Read the model definition and answer for the solid it produces. Units are mm, in the model's axes. A direction names the side the tool comes from. Coordinates: 2 decimals unless noted, no trailing zeros. Write each loop counter-clockwise with the first axis right and the second up, starting at its lowest first coordinate (ties: lowest second). Pieces come first, ordered by that corner, then holes. Notation, with made-up numbers: (79.5, 77.25) -> (116.5, 77.25) arc R24 cw to (116.5, 113.25) -> close; hole circle Ø8 at (2.25, 66). An arc over 180 degrees is marked (long way). Write item = value, one per line. Start each with the question number.
1) A tool of negligible diameter and unlimited length cuts with its end or side. For faces 5 (the face through (-45, 2, 35.813)), 6 (the face through (-41.221, 2, 18)), 7 (the face through (-32.721, 3, 27)), from which of +Z, -Z, +X, -X, +Y, -Y can it reach the whole face along a straight path? Write none if from no direction.
2) Section A-A (y = 1.3) is taken. Determine the outline of the cut face in (x, z), plus the area to 3 significant figures.
3) For a pull along Z with two mould halves and no side action, classify faces 1 (the face through (-41, 3.5, 34)), 2 (the face through (-45, 2, 36.813)), 3 (the face through (-36, 2, 17.613)), 4 (the face through (-32.221, 2, 27)) as released by +Z, released by -Z, zero draft, split by the parting line, or undercut.
4) Flat-ended cylindrical pins translate along their axes: pin 1 Ø1.1 at (y, z) = (3, 27) entering from -X; pin 2 Ø1.2 at (y, z) = (1, 18) entering from -X; pin 3 Ø1 at (x, y) = (-48, 1) entering from -Z. Find the tip coordinate at first contact, or state that the pin passes through.
5) Section B-B (z = 30.75) is taken. Determine the outline of the cut face in (x, y).
6) Find the intervals of material crossed by line 1 along X through (y, z) = (2.85, 26.5); line 2 along X through (y, z) = (2.45, 33); line 3 along Y through (x, z) = (-50.5, 34.75), in increasing order. Write a range as from..to.
from build123d import *

# Parameters (mm, degrees)
SKETCH1_W           = 26.9
SKETCH1_H           = 19.2
BOSS_EXTRUDE1_DEPTH = 3.5
CUT_EXTRUDE3_DEPTH  = 3.5
SKETCH4_W           = 17.2
SKETCH4_H           = 1.5
CUT_EXTRUDE4_DEPTH  = 25.9
FILLET1_DEPTH       = 1
FILLET2_START       = 2.5
FILLET2_DEPTH       = 1
FILLET3_SIZE        = 8.5
FILLET3_SIZE_2      = 2
FILLET4_START       = 2.5
FILLET4_DEPTH       = 1
FILLET6_SIZE        = 10
FILLET6_SIZE_2      = 2.5
FILLET7_SIZE        = 2.5
FILLET7_SIZE_2      = 10
FILLET8_R           = 2
FILLET9_R           = 2


with BuildPart() as part:
    # Sketch1 → Boss-Extrude1 (new body)
    with BuildSketch(Plane(origin=(0, 0, 0), x_dir=(1, 0, 0), z_dir=(0, 1, 0))):
        with Locations((-44.670982611, -27.213166741)):
            Rectangle(SKETCH1_W, SKETCH1_H)
    extrude(amount=BOSS_EXTRUDE1_DEPTH)

    # Sketch2 → Cut-Extrude3 (cut)
    with BuildSketch(Plane(origin=(0, 3.5, 0), x_dir=(1, 0, 0), z_dir=(0, 1, 0))):
        Polygon((-58.120982611, -33.313166741), (-32.720982611, -33.313166741), (-32.720982611, -20.613166741), (-41.220982611, -20.613166741), (-41.220982611, -17.613166741), (-58.120982611, -17.613166741), align=None)
    extrude(amount=-CUT_EXTRUDE3_DEPTH, mode=Mode.SUBTRACT)

    # Sketch4 → Cut-Extrude4 (cut)
    with BuildSketch(Plane.ZY.offset(58.120982611)):
        with Locations((27.213166741, 1.75)):
            Rectangle(SKETCH4_W, SKETCH4_H)
    extrude(amount=-CUT_EXTRUDE4_DEPTH, mode=Mode.SUBTRACT)

    # Fillet1: read off the stored shape, not the designer's step
    # Fillet1 outline → Fillet1 (add)
    with BuildSketch(Plane(origin=(0, 0, 0), x_dir=(1, 0, 0), z_dir=(0, 1, 0))):
        with BuildLine():
            add(Edge.make_bspline(
                [(-47.720982611, -33.313166741), (-32.720982611, -33.313166741), (-32.720982611, -31.313166741)],
                knots=[0, 0, 0, 1, 1, 1], degree=2, weights=[1, 0.707106781, 1]))
            Line((-47.720982611, -33.313166741), (-32.720982611, -33.313166741))
            Line((-32.720982611, -33.313166741), (-32.720982611, -31.313166741))
        make_face()
    extrude(amount=FILLET1_DEPTH)

    # Fillet2: read off the stored shape, not the designer's step
    # Fillet2 outline → Fillet2 (add)
    with BuildSketch(Plane(origin=(0, 0, 0), x_dir=(1, 0, 0), z_dir=(0, 1, 0)).offset(FILLET2_START)):
        with BuildLine():
            add(Edge.make_bspline(
                [(-47.720982611, -33.313166741), (-32.720982611, -33.313166741), (-32.720982611, -31.313166741)],
                knots=[0, 0, 0, 1, 1, 1], degree=2, weights=[1, 0.707106781, 1]))
            Line((-47.720982611, -33.313166741), (-32.720982611, -33.313166741))
            Line((-32.720982611, -33.313166741), (-32.720982611, -31.313166741))
        make_face()
    extrude(amount=FILLET2_DEPTH)

    # Fillet3
    # a fillet whose section is not a circle: 8.5, 2 mm, written as the material it adds along each edge
    with BuildSketch(Plane(origin=(-32.720982611, 1, 20.613166741), x_dir=(-1, 0, 0), z_dir=(0, -1, 0))) as fillet3_piece_1:
        with BuildLine():
            Bezier((FILLET3_SIZE, 0), (0, 0), (0, -FILLET3_SIZE_2), weights=[1, 0.707106781, 1])
            Line((0, -FILLET3_SIZE_2), (0, 0))
            Line((0, 0), (FILLET3_SIZE, 0))
        make_face()
    extrude(amount=1)

    # Fillet4: read off the stored shape, not the designer's step
    # Fillet4 outline → Fillet4 (add)
    with BuildSketch(Plane(origin=(0, 0, 0), x_dir=(1, 0, 0), z_dir=(0, 1, 0)).offset(FILLET4_START)):
        with BuildLine():
            Line((-32.720982611, -20.613166741), (-41.220982611, -20.613166741))
            add(Edge.make_bspline(
                [(-41.220982611, -20.613166741), (-32.720982611, -20.613166741), (-32.720982611, -22.613166741)],
                knots=[0, 0, 0, 1, 1, 1], degree=2, weights=[1, 0.707106781, 1]))
            Line((-32.720982611, -22.613166741), (-32.720982611, -20.613166741))
        make_face()
    extrude(amount=FILLET4_DEPTH)

    # Fillet6
    # a fillet whose section is not a circle: 10, 2.5 mm, written as the material it takes off along each edge
    with BuildSketch(Plane(origin=(-58.120982611, 26, 33.313166741), x_dir=(1, 0, 0), z_dir=(0, -1, 0))) as fillet6_piece_1_section:
        with BuildLine():
            Bezier((FILLET6_SIZE, 0), (0, 0), (0, FILLET6_SIZE_2), weights=[1, 0.707106781, 1])
            Line((0, FILLET6_SIZE_2), (0, 0))
            Line((0, 0), (FILLET6_SIZE, 0))
        make_face()
    fillet6_piece_1 = extrude(amount=51, mode=Mode.PRIVATE)
    fillet6_piece_1 = split(fillet6_piece_1, bisect_by=Plane(origin=(-58.120982611, 2.5, 33.313166741), z_dir=(0, -1, 0)), keep=Keep.TOP, mode=Mode.PRIVATE)
    add(fillet6_piece_1, mode=Mode.SUBTRACT)

    # Fillet7
    # a fillet whose section is not a circle: 10, 2.5 mm, written as the material it takes off along each edge
    with BuildSketch(Plane(origin=(-58.120982611, 28.5, 33.313166741), x_dir=(0, 0, 1), z_dir=(0, -1, 0))) as fillet7_piece_1:
        with BuildLine():
            Bezier((FILLET7_SIZE, 0), (0, 0), (0, -FILLET7_SIZE_2), weights=[1, 0.707106781, 1])
            Line((0, -FILLET7_SIZE_2), (0, 0))
            Line((0, 0), (FILLET7_SIZE, 0))
        make_face()
    extrude(amount=51, mode=Mode.SUBTRACT)

    # Fillet8
    fillet8_edges = [part.edges().sort_by_distance(p)[0] for p in [
        (-41.220982611, 0.5, 20.613166741),
    ]]
    fillet(fillet8_edges, radius=FILLET8_R)

    # Fillet9
    fillet9_edges = [part.edges().sort_by_distance(p)[0] for p in [
        (-41.220982611, 3, 20.613166741),
    ]]
    fillet(fillet9_edges, radius=FILLET9_R)


solid = part.part
Answer key:
q1.face_5 = -X
q1.face_6 = -Z, -X, +Y, -Y
q1.face_7 = -X, +Y, -Y
q2.outline = (-58.12, 35.81) -> (-32.22, 35.81) -> (-32.22, 18.61) -> (-41.22, 18.61) -> (-41.22, 17.61) -> (-31.22, 17.61) -> (-31.22, 36.81) -> (-58.12, 36.81) -> close
q2.area = 54.1 mm^2
q3.face_1 = zero draft
q3.face_2 = released by +Z
q3.face_3 = released by -Z
q3.face_4 = undercut
q4.pin_1 = -32.72
q4.pin_2 = -41.22
q4.pin_3 = 33.31
q5.outline = (-32.72, 0) -> (-31.22, 0) -> (-31.22, 3.5) -> (-32.72, 3.5) -> (-32.72, 2.5) -> (-32.22, 2.5) -> (-32.22, 1) -> (-32.72, 1) -> close
q6.line_1 = -32.72..-31.22
q6.line_2 = -32.22..-31.22
q6.line_3 = 0..1, 2.5..3.5
